Model file for the job. Use its own axes, mm. Round coordinates to 2 decimals unless told otherwise and drop trailing zeros. Loops run counter-clockwise (first coordinate to the right, second up) from the corner with the lowest first, then second, coordinate; pieces in that order, holes last. Notation, with made-up numbers: M -28,-2.75 L 9,-2.75 A21 cw 9,2.25 Z; hole C 86,-39.75 d9. An arc over 180 degrees is marked long. Use a Markdown table: item, result. Add a question column.
Q1. Cut at B-B (x = 11). State how many separate pieces and enclosed holes the cut face has, plus the area to 3 significant figures.
Q2. Cut at C-C (y = 16.5). Give the cut face in (x, z), plus the area to 3 significant figures.
Q3. Probe line 1 (Y direction, x = 18, z = 260); line 2 (X direction, y = 20.5, z = 219); line 3 (X direction, y = 33.55, z = 329). List the from-to ranges inside material, lowest first. Write a range as from..to.
Q4. Pin check, flat tips, straight feed: pin 1 (5 mm diameter, centred on y = 27.5, z = 431.5, fed in from +X); pin 2 (9 mm diameter, centred on x = 11, z = 278, fed in from -Y). Stop position of each tip, or through.
Q5. Cut at A-A (z = 211.5). Give the cut face in (x, y), plus the area to 3 significant figures.
from build123d import *

# Parameters (mm, degrees)
F1_DEPTH = 505
F2_R     = 4
F2_R_2   = 2.5
F3_DEPTH = 2.001
F4_R     = 4
F5_DEPTH = 2.001


with BuildPart() as f1:
    # F0 (on Top) → F1 (new body)
    with BuildSketch(Plane.XY):
        with BuildLine():
            Line((0, 32.7), (0, 0))
            Line((0, 0), (2, 0))
            Line((2, 0), (2, 32.2))
            Line((2, 32.2), (20, 32.2))
            Line((20, 32.2), (20, 34.2))
            Line((20, 34.2), (1.5, 34.2))
            ThreePointArc((1.5, 34.2), (0.43934, 33.76066), (0, 32.7))
        make_face()
    extrude(amount=F1_DEPTH)

    # F2 (on face) → F3 (cut, through all)
    with BuildSketch(Plane.YZ.offset(2)):
        with Locations((7.5, 431)):
            Circle(F2_R)
        with Locations((7.5, 380)):
            Circle(F2_R)
        with Locations((7.5, 329)):
            Circle(F2_R)
        with Locations((7.5, 278)):
            Circle(F2_R)
        with Locations((7.5, 227)):
            Circle(F2_R)
        with Locations((7.5, 176)):
            Circle(F2_R)
        with Locations((7.5, 125)):
            Circle(F2_R)
        with Locations((7.5, 74)):
            Circle(F2_R)
        with Locations((9, 12)):
            Circle(F2_R_2)
        with Locations((9, 493)):
            Circle(F2_R_2)
    extrude(amount=-F3_DEPTH, mode=Mode.SUBTRACT)

    # F4 (on face) → F5 (cut, through all)
    with BuildSketch(Plane.XZ.offset(-32.2)):
        with Locations((11, 74)):
            Circle(F4_R)
        with Locations((11, 125)):
            Circle(F4_R)
        with Locations((11, 12)):
            Circle(F4_R)
        with Locations((11, 176)):
            Circle(F4_R)
        with Locations((11, 227)):
            Circle(F4_R)
        with Locations((11, 278)):
            Circle(F4_R)
        with Locations((11, 329)):
            Circle(F4_R)
        with Locations((11, 380)):
            Circle(F4_R)
        with Locations((11, 431)):
            Circle(F4_R)
        with Locations((11, 493)):
            Circle(F4_R)
    extrude(amount=-F5_DEPTH, mode=Mode.SUBTRACT)


solid = f1.part
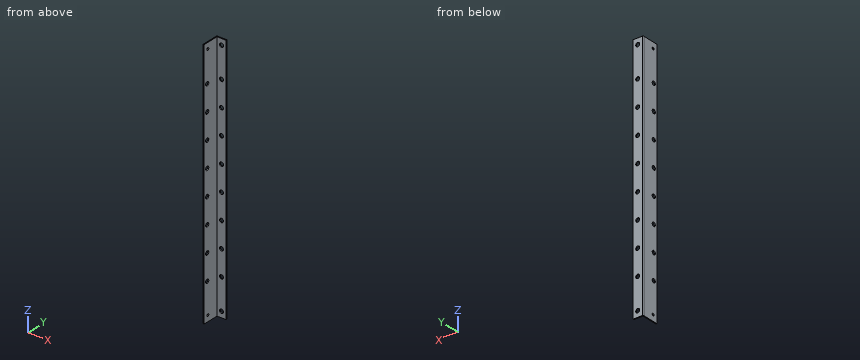
Checked values:
| question | item | result |
|---|---|---|
| 1 | separate pieces | 11 |
| 1 | enclosed holes | 0 |
| 1 | area | 850 mm^2 |
| 2 | outline | M 0,0 L 2,0 L 2,505 L 0,505 Z |
| 2 | area | 1,010 mm^2 |
| 3 | line 1 | y = 32.2..34.2 |
| 3 | line 2 | x = 0..2 |
| 3 | line 3 | x = 0.26..7, 15..20 |
| 4 | pin 1 | stops at x = 2 |
| 4 | pin 2 | stops at y = 32.2 |
| 5 | outline | M 0,0 L 2,0 L 2,32.2 L 20,32.2 L 20,34.2 L 1.5,34.2 A1.5 ccw 0,32.7 Z |
| 5 | area | 104 mm^2 |
